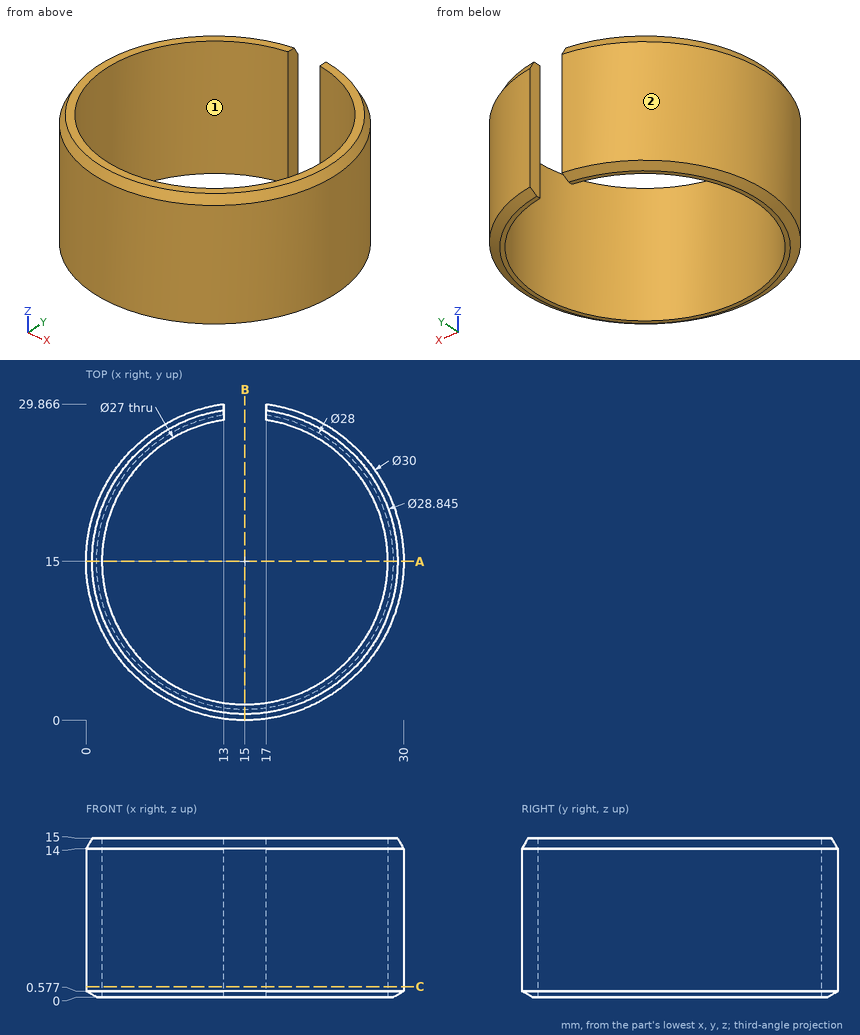
Answer from the drawing. Dimensions are ordinates in mm from the lowest x, y and z of the part. Give positions to 0.01 mm unless a question says otherwise; leave off trailing zeros. Order: outer loops, then holes, each group sorted by start corner. A loop starts at its lowest first (then second) coordinate and runs counter-clockwise, first axis right, second up. Notation, with made-up numbers: (-1.5, 41.5) - (27.5, 41.5) arc R21 ccw to (27.5, 51.5) - close; hole circle Ø7 at (-39, 22). An arc over 180 degrees is marked (long way). One line per item, written item: value. Start each with the question number.
1. Section C-C, the plane z = 1 is taken. Write down the section's boundary in (x, y), then the cut area to 3 significant figures.
2. For a pull along Y with two mould halves and no side action, classify the marked faces 1 and 2 as released by +Y, released by -Y, zero draft, split by the parting line, or undercut.
3. Section A-A, the plane y = 15 is taken. Write down the section's boundary in (x, z).
4. Consider line 1 (X direction, y = 15, z = 8.5); line 2 (Y direction, x = 15, z = 9); line 3 (Y direction, x = 7.5, z = 8.75) (1 decimal). Determine where each line is inside the solid, lowest interval first.
5. Section B-B, the plane x = 15 is taken. Write down the section's boundary in (y, z), then the cut area to 3 significant figures.
6. Each of these flat-tipped pins is pushed along its axis until it touches: pin 1 Ø12 at (x, y) = (24.5, 12) entering from +Z; pin 2 Ø8 at (x, z) = (24.5, 7) entering from +Y (1 decimal); pin 3 Ø1.2 at (y, z) = (29, 9.5) entering from -X; pin 4 Ø5 at (y, z) = (5.5, 8.5) entering from -X. Where does it stop, or does it pass through?
Filled sheet:
1. outline: (13, 28.35) - (13, 29.87) arc R15 ccw (long way) to (17, 29.87) - (17, 28.35) arc R13.5 cw (long way) to start
1. area: 128 mm²
2. face 1: undercut
2. face 2: split by the parting line
3. outline: (0, 0.58) - (1, 0) - (1.5, 0) - (1.5, 15) - (0.58, 15) - (0, 14) - close; (28.5, 0) - (29, 0) - (30, 0.58) - (30, 14) - (29.42, 15) - (28.5, 15) - close
4. line 1: 0 to 1.5, 28.5 to 30
4. line 2: 0 to 1.5
4. line 3: 2 to 3.8, 26.2 to 28
5. outline: (0, 0.58) - (1, 0) - (1.5, 0) - (1.5, 15) - (0.58, 15) - (0, 14) - close
5. area: 21.9 mm²
6. pin 1: z = 15
6. pin 2: y = 29
6. pin 3: x = 8.26
6. pin 4: x = 1.73
